Here's how the part is built. I have some questions about the finished solid (model axes, mm). A direction names the side the tool comes from. Coordinates: 2 decimals unless noted, no trailing zeros. Write each loop counter-clockwise with the first axis right and the second up, starting at its lowest first coordinate (ties: lowest second). Pieces come first, ordered by that corner, then holes. Notation, with made-up numbers: (41.25, 76.5) -> (79.25, 76.5) arc R20 cw to (79.25, 111.5) -> close; hole circle Ø10 at (24.25, 24). An arc over 180 degrees is marked (long way). Use a Markdown table: item, result. Add a question column.
Item 1: Imagine slicing it at C-C, the plane z = 18. Write out the boundary of the cut face in (x, y).
Item 2: If I drill on line 1 along Y through (x, z) = (0, 2.75); line 2 along X through (y, z) = (-6.75, 15); line 3 along X through (y, z) = (-5, 1.6), over which ranges is the centre line in solid material (lowest first)? Write a range as from..to.
Item 3: Will these pins go through, and if not, where does the flat tip stop? pin 1 Ø16.5 at (y, z) = (0, 35) entering from -X; pin 2 Ø5.5 at (x, y) = (0, -5) entering from +Z.
Item 4: Imagine slicing it at B-B, the plane y = 0. Write out the boundary of the cut face in (x, z), and give its area (3 significant figures).
Item 5: Imagine slicing it at A-A, the plane x = -5. Write out the boundary of the cut face in (y, z).
Item 6: On a 3-axis mill with a long thin cutter (end or side, diameter ignored), from which of +Z, -Z, +X, -X, +Y, -Y can I reach the whole of each face in a straight line? I mean faces 1 (the flat face through (0, 0, 5)), 2 (the flat face through (-25.71, 0, 19)), 3 (the cylindrical face through (-24.231, 2.255, 24.847)). Say none if no direction works.
Item 7: If we mould it in two halves opening along X, with no side actions, what happens to faces 4 (the flat face through (25.71, 0, 24)), 5 (the flat face through (22.71, 0, 27)), 6 (the flat face through (0, 0, 0))? For each: pulls with the +X half, pulls with the -X half, needs draft (parallel to the pull), parting line crosses it, or undercut.
Item 8: Imagine slicing it at D-D, the plane y = -6. Write out the boundary of the cut face in (x, z), and give its area (3 significant figures).
```python
from build123d import *

# Parameters (mm, degrees)
SKETCH1_W           = 51.42
SKETCH1_H           = 28
BOSS_EXTRUDE1_DEPTH = 5
SKETCH3_W           = 3
SKETCH3_H           = 28
BOSS_EXTRUDE2_DEPTH = 30
BOSS_EXTRUDE4_DEPTH = 3
SKETCH6_R           = 10.4
CUT_EXTRUDE1_DEPTH  = 4
BOSS_EXTRUDE5_START = -3
BOSS_EXTRUDE5_DEPTH = 3
SKETCH8_R           = 1.75
CUT_EXTRUDE2_DEPTH  = 10


with BuildPart() as part:
    # Sketch1 → Boss-Extrude1 (new body)
    with BuildSketch(Plane.XY):
        Rectangle(SKETCH1_W, SKETCH1_H)
    extrude(amount=BOSS_EXTRUDE1_DEPTH)

    # Sketch3 → Boss-Extrude2 (add)
    with BuildSketch(Plane.XY.offset(5)):
        with Locations((-24.21, 0)):
            Rectangle(SKETCH3_W, SKETCH3_H)
        with Locations((24.21, 0)):
            Rectangle(SKETCH3_W, SKETCH3_H)
    extrude(amount=BOSS_EXTRUDE2_DEPTH)

    # Sketch5 → Boss-Extrude4 (add)
    with BuildSketch(Plane.ZY.offset(25.71)):
        with BuildLine():
            Line((35, -14), (35, 14))
            ThreePointArc((35, 14), (49, 0), (35, -14))
        make_face()
    extrude(amount=-BOSS_EXTRUDE4_DEPTH)

    # Sketch6 → Cut-Extrude1 (cut)
    with BuildSketch(Plane.ZY.offset(25.71)):
        with Locations(Location((35, 0, 0), (0, 0, 270))):
            Circle(SKETCH6_R)
    extrude(amount=-CUT_EXTRUDE1_DEPTH, mode=Mode.SUBTRACT)

    # Sketch7 → Boss-Extrude5 (add)
    with BuildSketch(Plane(origin=(25.71, 0, 0), x_dir=(0, 0, -1), z_dir=(1, 0, 0)).offset(BOSS_EXTRUDE5_START)):
        with BuildLine():
            Line((-35, 14), (-35, -14))
            ThreePointArc((-35, -14), (-49, 0), (-35, 14))
        make_face()
    extrude(amount=BOSS_EXTRUDE5_DEPTH)

    # Sketch8 → Cut-Extrude2 (cut)
    with BuildSketch(Plane(origin=(0, 0, 0), x_dir=(-1, 0, 0), z_dir=(0, 0, -1))):
        with Locations((0, 5)):
            Circle(SKETCH8_R)
        with Locations((-5, 0)):
            Circle(SKETCH8_R)
        with Locations(Location((5, 0, 0), (0, 0, 180))):
            Circle(SKETCH8_R)
        with Locations(Location((0, -5, 0), (0, 0, 180))):
            Circle(SKETCH8_R)
    extrude(amount=-CUT_EXTRUDE2_DEPTH, mode=Mode.SUBTRACT)


solid = part.part
```
Ans:
| question | item | result |
|---|---|---|
| 1 | outline | (-25.71, -14) -> (-22.71, -14) -> (-22.71, 14) -> (-25.71, 14) -> close; (22.71, -14) -> (25.71, -14) -> (25.71, 14) -> (22.71, 14) -> close |
| 2 | line 1 | y = -14..-6.75, -3.25..3.25, 6.75..14 |
| 2 | line 2 | x = -25.71..-22.71, 22.71..25.71 |
| 2 | line 3 | x = -25.71..-1.75, 1.75..25.71 |
| 3 | pin 1 | stops at x = 22.71 |
| 3 | pin 2 | stops at z = 5 |
| 4 | outline | (-25.71, 0) -> (-6.75, 0) -> (-6.75, 5) -> (-22.71, 5) -> (-22.71, 24.6) -> (-25.71, 24.6) -> close; (-25.71, 45.4) -> (-22.71, 45.4) -> (-22.71, 49) -> (-25.71, 49) -> close; (-3.25, 0) -> (3.25, 0) -> (3.25, 5) -> (-3.25, 5) -> close; (6.75, 0) -> (25.71, 0) -> (25.71, 49) -> (22.71, 49) -> (22.71, 5) -> (6.75, 5) -> close |
| 4 | area | 424 mm^2 |
| 5 | outline | (-14, 0) -> (-1.75, 0) -> (-1.75, 5) -> (-14, 5) -> close; (1.75, 0) -> (14, 0) -> (14, 5) -> (1.75, 5) -> close |
| 6 | face 1 | +Z, +Y, -Y |
| 6 | face 2 | +Z, -Z, -X, +Y, -Y |
| 6 | face 3 | -X |
| 7 | face 4 | pulls with the +X half |
| 7 | face 5 | undercut |
| 7 | face 6 | needs draft |
| 8 | outline | (-25.71, 0) -> (-1.44, 0) -> (-1.44, 5) -> (-22.71, 5) -> (-22.71, 26.51) -> (-25.71, 26.51) -> close; (-25.71, 43.49) -> (-22.71, 43.49) -> (-22.71, 47.65) -> (-25.71, 47.65) -> close; (1.44, 0) -> (25.71, 0) -> (25.71, 47.65) -> (22.71, 47.65) -> (22.71, 5) -> (1.44, 5) -> close |
| 8 | area | 448 mm^2 |
